from build123d import *

# Parameters (mm, degrees)
SKETCH1_R                 = 4
BOSS_EXTRUDE1_DEPTH       = 26.35
M4X0_7_TAPPED_HOLE1_D     = 3.3
M4X0_7_TAPPED_HOLE1_DEPTH = 15
M4X0_7_TAPPED_HOLE1_TIP   = 0.991420021
M4X0_7_TAPPED_HOLE2_D     = 3.3
M4X0_7_TAPPED_HOLE2_DEPTH = 15
M4X0_7_TAPPED_HOLE2_TIP   = 0.991420021


with BuildPart() as part:
    # Sketch1 → Boss-Extrude1 (new body, symmetric)
    with BuildSketch(Plane(origin=(0, 0, 0), x_dir=(1, 0, 0), z_dir=(0, 1, 0))):
        Circle(SKETCH1_R)
    extrude(amount=BOSS_EXTRUDE1_DEPTH, both=True)

    # M4x0.7 Tapped Hole1
    with Locations(Plane(origin=(0, 26.35, 0), x_dir=(1, 0, 0), z_dir=(0, 1, 0))):
        with Locations((0, 0)):
            Hole(M4X0_7_TAPPED_HOLE1_D / 2, depth=M4X0_7_TAPPED_HOLE1_DEPTH)
            with Locations((0, 0, -(M4X0_7_TAPPED_HOLE1_DEPTH + M4X0_7_TAPPED_HOLE1_TIP / 2))):  # 118° drill point
                Cone(0, M4X0_7_TAPPED_HOLE1_D / 2, M4X0_7_TAPPED_HOLE1_TIP, mode=Mode.SUBTRACT)

    # M4x0.7 Tapped Hole2
    with Locations(Plane(origin=(0, -26.35, 0), x_dir=(-1, 0, 0), z_dir=(0, -1, 0))):
        with Locations((0, 0)):
            Hole(M4X0_7_TAPPED_HOLE2_D / 2, depth=M4X0_7_TAPPED_HOLE2_DEPTH)
            with Locations((0, 0, -(M4X0_7_TAPPED_HOLE2_DEPTH + M4X0_7_TAPPED_HOLE2_TIP / 2))):  # 118° drill point
                Cone(0, M4X0_7_TAPPED_HOLE2_D / 2, M4X0_7_TAPPED_HOLE2_TIP, mode=Mode.SUBTRACT)


solid = part.part
Geometry: final body of the model. Coordinates: model frame, mm. A direction names the side the tool comes from. Coordinates: 2 decimals unless noted, no trailing zeros. Order: outer loops, then holes, each group sorted by start corner. A loop starts at its lowest first (then second) coordinate and runs counter-clockwise, first axis right, second up. Notation, with made-up numbers: (22.25, -13) - (80.25, -13) arc R19 cw to (80.25, 0) - close; hole circle Ø10 at (50, 56.5). An arc over 180 degrees is marked (long way). Use one line per item in the form item = value.
1) Mould query, pull axis X, two halves, no side actions, for faces 4 (the face through (2, 26.35, 0)), 5 (the face through (-0.867, 0.369, 3.905)), 6 (the face through (0.26, 10.53, 0.11)). Classes: +X half, -X half, draft (parallel to the pull), parting line (faces both ways), or undercut.
Solutions:
face_4 = draft
face_5 = parting line
face_6 = undercut
2) Pin query (flat end, axial travel): pin 1 (2 mm diameter, centred on x = 2, y = 12.5, fed in from -Z); pin 2 (4 mm diameter, centred on y = 16.5, z = -3, fed in from +X); pin 3 (1 mm diameter, centred on y = -10, z = 1.5, fed in from -X). Return the tip coordinate at first contact, or that it passes through.
Solutions:
pin_1 = -3.87
pin_2 = 3.87
pin_3 = -3.87
3) Section C-C (x = -3). Return loops of the section in (y, z), then the cut area to 3 significant figures.
Solutions:
outline = (-26.35, -2.65) - (26.35, -2.65) - (26.35, 2.65) - (-26.35, 2.65) - close
area = 279 mm^2
4) Section A-A (y = 7). Return loops of the section in (x, z).
Solutions:
outline = circle Ø8 at (0, 0)
5) Set-up query: faces 1 (the face through (-1.216, -18.745, -1.115)), 2 (the face through (2, -26.35, 0)), 3 (the face through (1.216, 18.745, -1.115)). Return all of +Z, -Z, +X, -X, +Y, -Y with unobstructed straight access to the full face (end or side cutting, diameter ignored); none if empty.
Solutions:
face_1 = -Y
face_2 = +Z, -Z, +X, -X, -Y
face_3 = +Y
6) Ray query, L1, parallel to Z at x = 0, y = 17; L2, parallel to X at y = 22, z = 1.5; L3, parallel to Z at x = -1.5, y = 3. Return the intervals inside material, ascending.
Solutions:
L1 = -4 to -1.65, 1.65 to 4
L2 = -3.71 to -0.69, 0.69 to 3.71
L3 = -3.71 to 3.71
7) Section B-B (y = 13.5). Return loops of the section in (x, z).
Solutions:
outline = circle Ø8 at (0, 0); hole circle Ø3.3 at (0, 0)
